Model file for the job. Use its own axes, mm. A direction names the side the tool comes from. Round coordinates to 2 decimals unless told otherwise and drop trailing zeros. Order: outer loops, then holes, each group sorted by start corner. A loop starts at its lowest first (then second) coordinate and runs counter-clockwise, first axis right, second up. Notation, with made-up numbers: (9, 46) - (40, 46) arc R16 ccw to (40, 52) - close; hole circle Ø5 at (70, 7.25). An arc over 180 degrees is marked (long way). Write item = value, one per line. Start each with the question number.
from build123d import *

# Parameters (mm, degrees)
ESBO_O1_R                 = 9.1
RESSALTO_EXTRUS_O1_DEPTH  = 3
ESBO_O2_R                 = 5.5
RESSALTO_EXTRUS_O2_DEPTH  = 80
RESSALTO_EXTRUS_O3_DEPTH  = 10
FURO_ROSCADO_DE_M21_D     = 1.6
FURO_ROSCADO_DE_M21_DEPTH = 10
FURO_ROSCADO_DE_M21_TIP   = 0.480688495


with BuildPart() as part:
    # Esboço1 → Ressalto-extrusão1 (new body)
    with BuildSketch(Plane.XY):
        Circle(ESBO_O1_R)
    extrude(amount=RESSALTO_EXTRUS_O1_DEPTH)

    # Esboço2 → Ressalto-extrusão2 (add)
    with BuildSketch(Plane.XY.offset(3)):
        Circle(ESBO_O2_R)
    extrude(amount=RESSALTO_EXTRUS_O2_DEPTH)

    # Esboço3 → Ressalto-extrusão3 (add)
    with BuildSketch(Plane.XY.offset(83)):
        with BuildLine():
            Line((-5.5, 0), (5.5, 0))
            ThreePointArc((5.5, 0), (0, -5.5), (-5.5, 0))
        make_face()
    extrude(amount=RESSALTO_EXTRUS_O3_DEPTH)

    # Furo roscado de M21
    with Locations(Plane.XY.offset(93)):
        with Locations((-2.474873734, -2.474873734), (2.474873734, -2.474873734)):
            Hole(FURO_ROSCADO_DE_M21_D / 2, depth=FURO_ROSCADO_DE_M21_DEPTH)
            with Locations((0, 0, -(FURO_ROSCADO_DE_M21_DEPTH + FURO_ROSCADO_DE_M21_TIP / 2))):  # 118° drill point
                Cone(0, FURO_ROSCADO_DE_M21_D / 2, FURO_ROSCADO_DE_M21_TIP, mode=Mode.SUBTRACT)


solid = part.part
Item 1: Saw through at D-D, the plane y = 7. Give the cut face in (x, z).
Item 2: Drop flat-ended pins along their axis: pin 1 (1.5 mm diameter, centred on x = 0.5, z = 42.5, fed in from +Y); pin 2 (1.5 mm diameter, centred on x = 1, z = 52.5, fed in from -Y); pin 3 (5.5 mm diameter, centred on x = 1.5, y = 3.5, fed in from +Z). Give the stop position or say it passes through.
Item 3: Saw through at A-A, the plane x = 0. Give the cut face in (y, z), then the cut area to 3 significant figures.
Item 4: Probe L1, parallel to Z at x = -2.5, y = -8; L2, parallel to Z at x = -2.5, y = 0.25; L3, parallel to Y at x = 0.25, z = 10. List the from-to ranges inside material, lowest first.
Item 5: Mould opens along X. For faces 1 (the face through (-0.716, -5.453, 47.37)), 2 (the face through (-2.411, -2.598, 82.603)), 3 (the face through (0, -2, 93)) say: +X half, -X half, draft (parallel to the pull), parting line (faces both ways), or undercut.
Item 6: Saw through at B-B, the plane y = 1.5. Give the cut face in (x, z), then the cut area to 3 significant figures.
Item 7: Which spindle directions (+Z, -Z, +X, -X, +Y, -Y) get a long thin tool onto all of the face, cutting with end or side? Do faces 4 (the face through (0, 0, 0)), 5 (the face through (4, -4, 3)), 6 (the face through (0, 2, 83)). Say none if no direction does.
Item 8: Saw through at C-C, the plane z = 21.5. Give the cut face in (x, y).
Check sheet entries:
q1.outline = (-5.81, 0) - (5.81, 0) - (5.81, 3) - (-5.81, 3) - close
q2.pin_1 = 5.5
q2.pin_2 = -5.49
q2.pin_3 = 83
q3.outline = (-9.1, 0) - (9.1, 0) - (9.1, 3) - (5.5, 3) - (5.5, 83) - (0, 83) - (0, 93) - (-5.5, 93) - (-5.5, 3) - (-9.1, 3) - close
q3.area = 990 mm2
q4.L1 = 0 to 3
q4.L2 = 0 to 83
q4.L3 = -5.49 to 5.49
q5.face_1 = parting line
q5.face_2 = undercut
q5.face_3 = draft
q6.outline = (-8.98, 0) - (8.98, 0) - (8.98, 3) - (5.29, 3) - (5.29, 83) - (-5.29, 83) - (-5.29, 3) - (-8.98, 3) - close
q6.area = 900 mm2
q7.face_4 = -Z, +X, -X, +Y, -Y
q7.face_5 = +Z
q7.face_6 = +Z, +X, -X, +Y
q8.outline = circle Ø11 at (0, 0)
